```python
from build123d import *

# Parameters (mm, degrees)
SKETCH1_R           = 57.15
SKETCH1_R_2         = 14.2875
SKETCH1_R_3         = 7.9375
BOSS_EXTRUDE1_DEPTH = 6.35
CUT_EXTRUDE1_REACH  = 8.35
SKETCH4_R           = 2.54


with BuildPart() as part:
    # Sketch1 → Boss-Extrude1 (new body)
    with BuildSketch(Plane(origin=(0, 0, 0), x_dir=(0, 0, -1), z_dir=(1, 0, 0))):
        Circle(SKETCH1_R)
        Circle(SKETCH1_R_2, mode=Mode.SUBTRACT)
        with Locations((0, 44.45)):
            Circle(SKETCH1_R_3, mode=Mode.SUBTRACT)
        with Locations((26.127054464, 35.9608054)):
            Circle(SKETCH1_R_3, mode=Mode.SUBTRACT)
        with Locations((42.274462149, 13.7358054)):
            Circle(SKETCH1_R_3, mode=Mode.SUBTRACT)
        with Locations((42.274462149, -13.7358054)):
            Circle(SKETCH1_R_3, mode=Mode.SUBTRACT)
        with Locations((26.127054464, -35.9608054)):
            Circle(SKETCH1_R_3, mode=Mode.SUBTRACT)
        with Locations((0, -44.45)):
            Circle(SKETCH1_R_3, mode=Mode.SUBTRACT)
        with Locations((-26.127054464, -35.9608054)):
            Circle(SKETCH1_R_3, mode=Mode.SUBTRACT)
        with Locations((-42.274462149, -13.7358054)):
            Circle(SKETCH1_R_3, mode=Mode.SUBTRACT)
        with Locations((-42.274462149, 13.7358054)):
            Circle(SKETCH1_R_3, mode=Mode.SUBTRACT)
        with Locations((-26.127054464, 35.9608054)):
            Circle(SKETCH1_R_3, mode=Mode.SUBTRACT)
    extrude(amount=BOSS_EXTRUDE1_DEPTH)

    # Sketch4 → Cut-Extrude1 (cut, up to next)
    with BuildSketch(Plane.ZY, mode=Mode.PRIVATE) as cut_extrude1_sk1:
        with Locations((-11.90625, -20.622229928)):
            Circle(SKETCH4_R)
    cut_extrude1_tool1 = extrude(cut_extrude1_sk1.sketch, amount=-CUT_EXTRUDE1_REACH, mode=Mode.PRIVATE) & part.part
    add(cut_extrude1_tool1.solids().sort_by_distance((0, -20.62223, -11.90625))[0], mode=Mode.SUBTRACT)
    # Sketch4 → Cut-Extrude1 (cut, up to next)
    with BuildSketch(Plane.ZY, mode=Mode.PRIVATE) as cut_extrude1_sk2:
        with Locations((-23.8125, 0)):
            Circle(SKETCH4_R)
    cut_extrude1_tool2 = extrude(cut_extrude1_sk2.sketch, amount=-CUT_EXTRUDE1_REACH, mode=Mode.PRIVATE) & part.part
    add(cut_extrude1_tool2.solids().sort_by_distance((0, 0, -23.8125))[0], mode=Mode.SUBTRACT)
    # Sketch4 → Cut-Extrude1 (cut, up to next)
    with BuildSketch(Plane.ZY, mode=Mode.PRIVATE) as cut_extrude1_sk3:
        with Locations((-11.90625, 20.622229928)):
            Circle(SKETCH4_R)
    cut_extrude1_tool3 = extrude(cut_extrude1_sk3.sketch, amount=-CUT_EXTRUDE1_REACH, mode=Mode.PRIVATE) & part.part
    add(cut_extrude1_tool3.solids().sort_by_distance((0, 20.62223, -11.90625))[0], mode=Mode.SUBTRACT)
    # Sketch4 → Cut-Extrude1 (cut, up to next)
    with BuildSketch(Plane.ZY, mode=Mode.PRIVATE) as cut_extrude1_sk4:
        with Locations((11.90625, 20.622229928)):
            Circle(SKETCH4_R)
    cut_extrude1_tool4 = extrude(cut_extrude1_sk4.sketch, amount=-CUT_EXTRUDE1_REACH, mode=Mode.PRIVATE) & part.part
    add(cut_extrude1_tool4.solids().sort_by_distance((0, 20.62223, 11.90625))[0], mode=Mode.SUBTRACT)
    # Sketch4 → Cut-Extrude1 (cut, up to next)
    with BuildSketch(Plane.ZY, mode=Mode.PRIVATE) as cut_extrude1_sk5:
        with Locations((23.8125, 0)):
            Circle(SKETCH4_R)
    cut_extrude1_tool5 = extrude(cut_extrude1_sk5.sketch, amount=-CUT_EXTRUDE1_REACH, mode=Mode.PRIVATE) & part.part
    add(cut_extrude1_tool5.solids().sort_by_distance((0, 0, 23.8125))[0], mode=Mode.SUBTRACT)
    # Sketch4 → Cut-Extrude1 (cut, up to next)
    with BuildSketch(Plane.ZY, mode=Mode.PRIVATE) as cut_extrude1_sk6:
        with Locations((11.90625, -20.622229928)):
            Circle(SKETCH4_R)
    cut_extrude1_tool6 = extrude(cut_extrude1_sk6.sketch, amount=-CUT_EXTRUDE1_REACH, mode=Mode.PRIVATE) & part.part
    add(cut_extrude1_tool6.solids().sort_by_distance((0, -20.62223, 11.90625))[0], mode=Mode.SUBTRACT)


solid = part.part
```
Geometry check sheet. Reference: the model listing, model coordinates, mm. Coordinates: 2 decimals unless noted, no trailing zeros. Order: outer loops, then holes, each group sorted by start corner. A loop starts at its lowest first (then second) coordinate and runs counter-clockwise, first axis right, second up. Notation, with made-up numbers: M 27.5,-18.5 L 76.5,-18.5 A22 ccw 76.5,13.5 Z; hole C 8.25,33.5 d9. An arc over 180 degrees is marked long. One line per question, with ' | ' between items. Start each with the question number.
Item 1: Cross-section at C-C on x = 5.25. State how many separate pieces and enclosed holes the cut face has, then the cut area to 3 significant figures.
Item 2: Draft check along Y on faces 1 (the cylindrical face through (3.13, -23.1, -12.46)), 2 (the flat face through (0, -12, -12)), 3 (the cylindrical face through (3.131, 2.513, 57.095)). Enter one of: pulls with the +Y half, pulls with the -Y half, needs draft (parallel to the pull), parting line crosses it, or undercut.
Item 3: Material ranges on L1, parallel to Y at x = 4, z = 0; L2, parallel to Z at x = 1.5, y = -42; L3, parallel to Z at x = 3.75, y = 19, recorded low to high. Write a range as [from, to].
Item 4: Cross-section at A-A on z = 0. Enter the section's corners in (x, y).
Item 5: Gauge pin test, flat ends, axial feed: pin 1 (20.5 mm diameter, centred on y = -13.74, z = 42.27, fed in from -X); pin 2 (2 mm diameter, centred on x = 4, y = 22.5, fed in from +Z); pin 3 (1 mm diameter, centred on x = 3, z = -2.5, fed in from +Y) (3 decimals); pin 4 (2 mm diameter, centred on x = 5, z = -23, fed in from +Y). Record the tip position at first contact, or that the pin passes through.
Item 6: Cross-section at B-B on y = 0. Enter the section's corners in (x, z), then the cut area to 3 significant figures.
Item 7: Cross-section at D-D on z = -37. Enter the section's corners in (x, y), then the cut area to 3 significant figures.
Findings:
1) separate pieces: 1 | enclosed holes: 17 | area: 7,520 mm²
2) face 1: undercut | face 2: needs draft | face 3: parting line crosses it
3) L1: y = [-57.15, -52.39], [-36.51, -14.29], [14.29, 36.51], [52.39, 57.15] | L2: z = [-38.76, -31.28], [-20.98, -7.55], [7.55, 20.98], [31.28, 38.76] | L3: z = [-53.9, -48.22], [-36.33, -13.86], [-9.95, 9.95], [13.86, 36.33], [48.22, 53.9]
4) outline: M 0,-57.15 L 6.35,-57.15 L 6.35,-52.39 L 0,-52.39 Z; M 0,-36.51 L 6.35,-36.51 L 6.35,-14.29 L 0,-14.29 Z; M 0,14.29 L 6.35,14.29 L 6.35,36.51 L 0,36.51 Z; M 0,52.39 L 6.35,52.39 L 6.35,57.15 L 0,57.15 Z
5) pin 1: stops at x = 0 | pin 2: stops at z = 52.95 | pin 3: stops at y = 57.115 | pin 4: stops at y = 52.75
6) outline: M 0,-57.15 L 6.35,-57.15 L 6.35,-26.35 L 0,-26.35 Z; M 0,-21.27 L 6.35,-21.27 L 6.35,-14.29 L 0,-14.29 Z; M 0,14.29 L 6.35,14.29 L 6.35,21.27 L 0,21.27 Z; M 0,26.35 L 6.35,26.35 L 6.35,57.15 L 0,57.15 Z | area: 480 mm²
7) outline: M 0,-43.56 L 6.35,-43.56 L 6.35,-19.67 L 0,-19.67 Z; M 0,-7.8 L 6.35,-7.8 L 6.35,7.8 L 0,7.8 Z; M 0,19.67 L 6.35,19.67 L 6.35,43.56 L 0,43.56 Z | area: 402 mm²
